Geometry check sheet. Reference: drawing and pictorial views, mm from the part's lowest x, y, z. Give positions to 0.01 mm unless a question says otherwise; leave off trailing zeros. Write each loop counter-clockwise with the first axis right and the second up, starting at its lowest first coordinate (ties: lowest second). Pieces come first, ordered by that corner, then holes. Notation, with made-up numbers: (77.5, -24.75) -> (126.5, -24.75) arc R6 cw to (126.5, -19.75) -> close; hole circle Ø5 at (-4, 20). An arc over 180 degrees is marked (long way). Return JSON: item names as keys, results as strings.
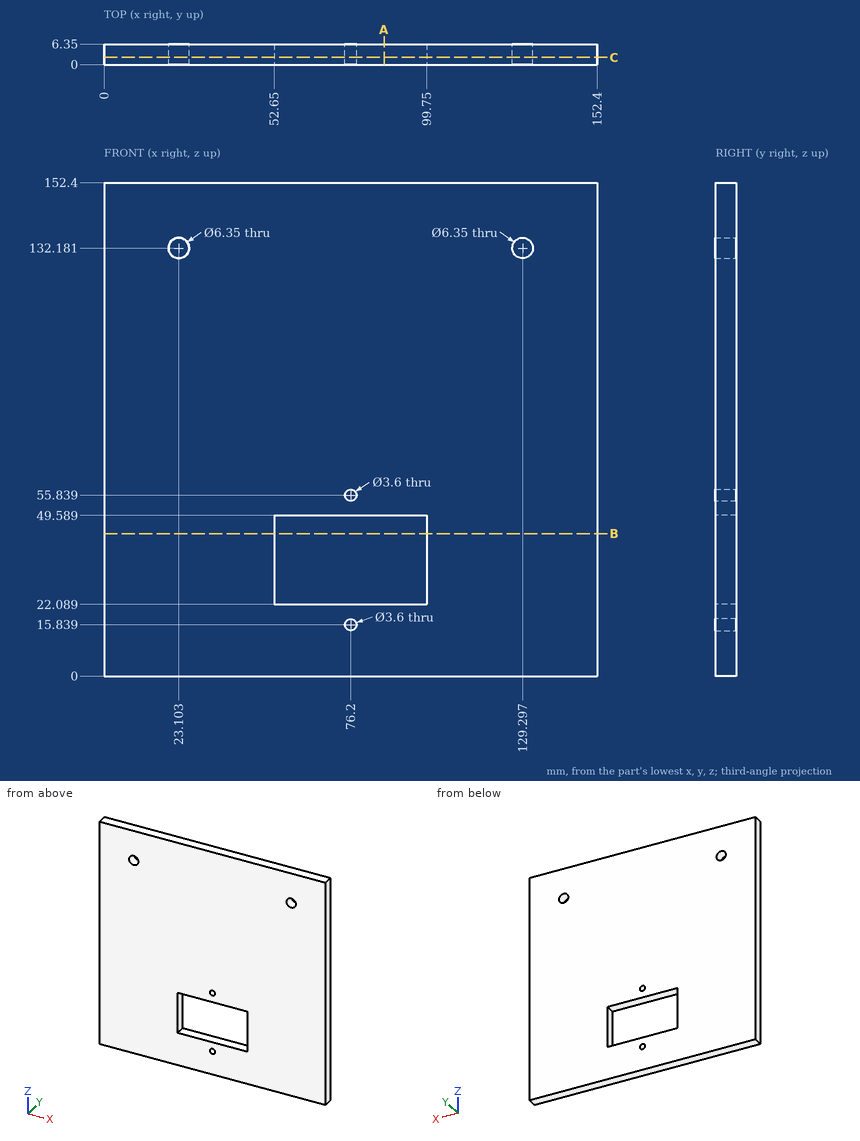
(1) Thickness scan on L1, parallel to Z at x = 76.2, y = 4.5; L2, parallel to X at y = 6, z = 35.5; L3, parallel to Z at x = 90, y = 5.75. Record the ranges inside material, lowest first.
Reply:
{"L1": "0 to 14.04, 17.64 to 22.09, 49.59 to 54.04, 57.64 to 152.4", "L2": "0 to 52.65, 99.75 to 152.4", "L3": "0 to 22.09, 49.59 to 152.4"}
(2) Cross-section at B-B on z = 44. Enter the section's corners in (x, y).
Reply:
{"outline": "(0, 0) -> (52.65, 0) -> (52.65, 6.35) -> (0, 6.35) -> close; (99.75, 0) -> (152.4, 0) -> (152.4, 6.35) -> (99.75, 6.35) -> close"}
(3) Cross-section at C-C on y = 2.25. Enter the section's corners in (x, z) (3 decimals).
Reply:
{"outline": "(0, 0) -> (152.4, 0) -> (152.4, 152.4) -> (0, 152.4) -> close; hole circle Ø6.35 at (23.103, 132.181); hole (52.65, 22.089) -> (99.75, 22.089) -> (99.75, 49.589) -> (52.65, 49.589) -> close; hole circle Ø3.6 at (76.2, 15.839); hole circle Ø3.6 at (76.2, 55.839); hole circle Ø6.35 at (129.297, 132.181)"}
(4) Cross-section at A-A on x = 86.5. Enter the section's corners in (y, z), then the cut area to 3 significant figures.
Reply:
{"outline": "(0, 0) -> (6.35, 0) -> (6.35, 22.09) -> (0, 22.09) -> close; (0, 49.59) -> (6.35, 49.59) -> (6.35, 152.4) -> (0, 152.4) -> close", "area": "793 mm^2"}
